from build123d import *

# Parameters (mm, degrees)
F0_W     = 30
F0_H     = 45
F1_DEPTH = 2
F2_W     = 7.129192
F2_H     = 6.062236
F2_R     = 2.40786
F3_DEPTH = 2.001
F4_R     = 2


with BuildPart() as f1:
    # F0 (on Front) → F1 (new body)
    with BuildSketch(Plane.XZ):
        with Locations((23.987818, 33.938015)):
            Rectangle(F0_W, F0_H)
    extrude(amount=F1_DEPTH)

    # F2 (on Front) → F3 (cut, through all)
    with BuildSketch(Plane.XZ):
        with Locations((12.552414, 53.406897)):
            Rectangle(F2_W, F2_H)
        with Locations((32.902706, 51.254064)):
            Circle(F2_R)
    extrude(amount=F3_DEPTH, mode=Mode.SUBTRACT)

    # F4
    f4_edges = [f1.edges().sort_by_distance(p)[0] for p in [
        (8.987818, -1, 50.375779),
        (16.11701, -1, 50.375779),
        (16.11701, -1, 56.438015),
        (38.987818, -1, 56.438015),
        (38.987818, -1, 11.438015),
        (8.987818, -1, 11.438015),
    ]]
    fillet(f4_edges, radius=F4_R)


solid = f1.part
The listing builds one solid part. Answer for the finished solid, in the listing's coordinates (mm). A direction names the side the tool comes from. Round coordinates to 2 decimals unless told otherwise and drop trailing zeros. Order: outer loops, then holes, each group sorted by start corner. A loop starts at its lowest first (then second) coordinate and runs counter-clockwise, first axis right, second up. Notation, with made-up numbers: M 24.25,89 L 58.25,89 A19 ccw 58.25,96 Z; hole C -16,78.5 d11. An arc over 180 degrees is marked long. Answer in a Markdown table with one row per item. Add a question column.
1) Which of the six approach directions +Z, -Z, +X, -X, +Y, -Y give full straight-line access (tool end or side, diameter ignored) to faces 4 (the face through (13, -1, 50.376)), 5 (the face through (38.988, -1, 34))?
2) The part is cut by section B-B on y = -1.1. Determine the outline of the cut face in (x, z).
3) Consider line 1 along Z through (x, y) = (11.5, -1); line 2 along X through (y, z) = (-1.45, 51); line 3 along X through (y, z) = (-0.4, 49.5). Determine where each line is inside the solid, lowest interval first. Write a range as from..to.
4) A flat-ended cylindrical pin translates along its axis: pin 1 Ø0.6 at (x, y) = (13, -0.5) entering from +Z. Find the tip coordinate at first contact, or state that the pin passes through.
5) The part is cut by section A-A on x = 34. Determine the outline of the cut face in (y, z).
6) The part is cut by section C-C on x = 13.5. Determine the outline of the cut face in (y, z).
7) Determine the mould class of faces 1 (the face through (38.39, -1.01, 12.01)), 2 (the face through (32.4, -1, 48.9)), 3 (the face through (24, -2, 34)) for opening direction Z: pulls with the +Z half, pulls with the -Z half, needs draft (parallel to the pull), parting line crosses it, or undercut.
Findings below:
| question | item | result |
|---|---|---|
| 1 | face 4 | +Z, -X, +Y, -Y |
| 1 | face 5 | +Z, -Z, +X, +Y, -Y |
| 2 | outline | M 8.99,13.44 A2 ccw 10.99,11.44 L 36.99,11.44 A2 ccw 38.99,13.44 L 38.99,54.44 A2 ccw 36.99,56.44 L 18.12,56.44 A2 ccw 16.12,54.44 L 16.12,52.38 A2 cw 14.12,50.38 L 10.99,50.38 A2 ccw 8.99,48.38 Z; hole C 32.9,51.25 d4.82 |
| 3 | line 1 | z = 11.44..50.38 |
| 3 | line 2 | x = 15.57..30.51, 35.3..38.99 |
| 3 | line 3 | x = 9.33..31.25, 34.55..38.99 |
| 4 | pin 1 | stops at z = 50.38 |
| 5 | outline | M -2,11.44 L 0,11.44 L 0,49.11 L -2,49.11 Z; M -2,53.4 L 0,53.4 L 0,56.44 L -2,56.44 Z |
| 6 | outline | M -2,11.44 L 0,11.44 L 0,50.38 L -2,50.38 Z |
| 7 | face 1 | pulls with the -Z half |
| 7 | face 2 | undercut |
| 7 | face 3 | needs draft |
